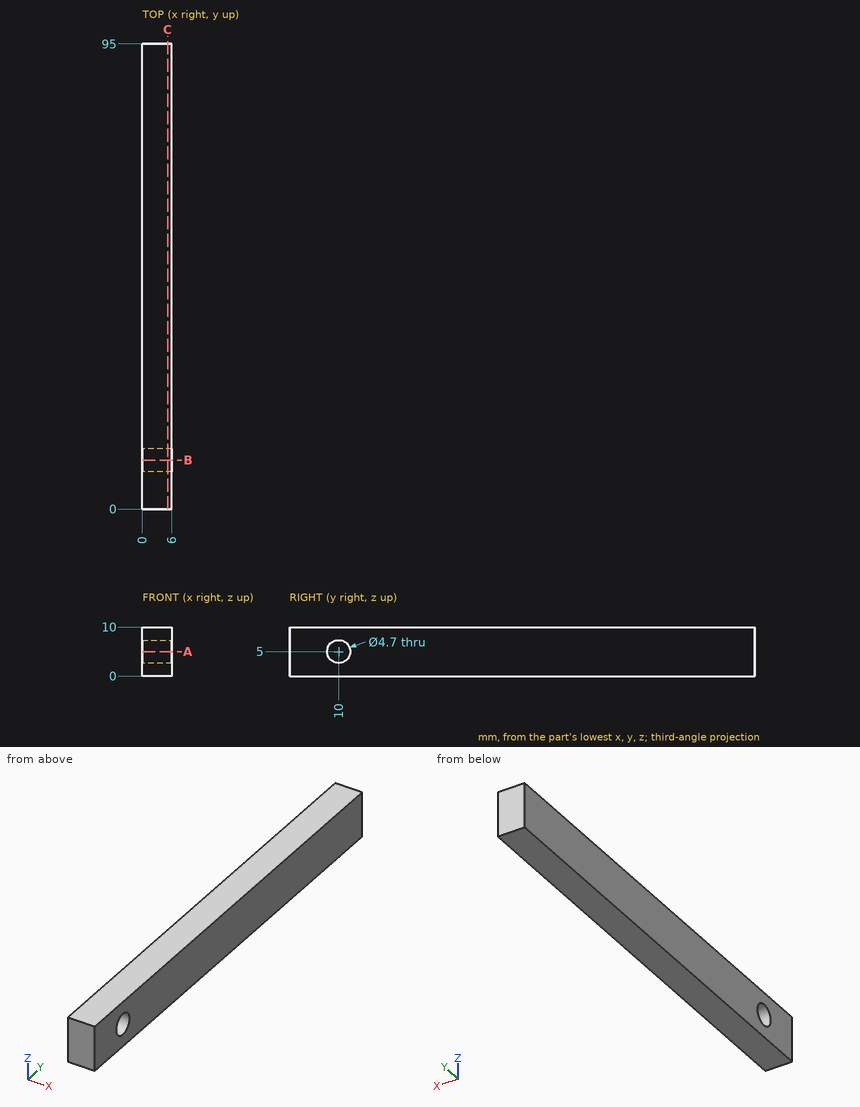
Check sheet for the drawn part. Datum: minimum x, y, z corner. Units: mm. Round coordinates to 2 decimals unless told otherwise and drop trailing zeros. Order: outer loops, then holes, each group sorted by start corner. A loop starts at its lowest first (then second) coordinate and runs counter-clockwise, first axis right, second up. Notation, with made-up numbers: (8, 40.25) -> (26, 40.25) arc R8 ccw to (26, 49.25) -> close; hole circle Ø5 at (51.25, 19). An arc over 180 degrees is marked (long way). Return JSON: item names as keys, results as strings. Group by question number.
Q1. Section check C-C, the plane x = 5.15. Record the boundary of the cut face in (y, z).
Q2. Material ranges on probe 1 along Y at (x, z) = (3.9, 5); probe 2 along Y at (x, z) = (3.35, 6.75), recorded low to high. Write a range as from..to.
Q3. Section check A-A, the plane z = 5. Record the boundary of the cut face in (x, y), plus the area to 3 significant figures.
Q4. Section check B-B, the plane y = 10. Record the boundary of the cut face in (x, z), plus the area to 3 significant figures.
Numbers:
{
 "1": {"outline": "(0, 0) -> (95, 0) -> (95, 10) -> (0, 10) -> close; hole circle Ø4.7 at (10, 5)"},
 "2": {"probe 1": "0..7.65, 12.35..95", "probe 2": "0..8.43, 11.57..95"},
 "3": {"outline": "(0, 0) -> (6, 0) -> (6, 7.65) -> (0, 7.65) -> close; (0, 12.35) -> (6, 12.35) -> (6, 95) -> (0, 95) -> close", "area": "542 mm^2"},
 "4": {"outline": "(0, 0) -> (6, 0) -> (6, 2.65) -> (0, 2.65) -> close; (0, 7.35) -> (6, 7.35) -> (6, 10) -> (0, 10) -> close", "area": "31.8 mm^2"}
}
